Study the drawing (mm; zero at the part's minimum x, y, z) and answer. A direction names the side the tool comes from. Round coordinates to 2 decimals unless told otherwise and drop trailing zeros. Loops run counter-clockwise (first coordinate to the right, second up) from the corner with the lowest first, then second, coordinate; pieces in that order, holes last. Notation, with made-up numbers: M 76.25,72.5 L 90.25,72.5 A22 ccw 90.25,93.5 Z; hole C -12,49 d2. An arc over 180 degrees is marked long. Put each result on its own line as item: value. Start each with the question number.
(1) Which of the six approach directions +Z, -Z, +X, -X, +Y, -Y give full straight-line access (tool end or side, diameter ignored) to the marked faces 4 and 5?
(2) Flat-ended cylindrical pins translate along their axes: P1, Ø3.5, axis at x = 4.5, z = 35.5, coming from the -Y side; P2, Ø13, axis at y = 15, z = 15, coming from the -X side; P3, Ø3.5, axis at x = 4.5, z = 36, coming from the +Y side. Find the tip coordinate at first contact, or state that the pin passes through.
(3) Straight lines are drawn through the part: line 1 (Z direction, x = 4.25, y = 15) (3 decimals); line 2 (Y direction, x = 2.25, z = 15); line 3 (Y direction, x = 3.25, z = 33). For each, find the intervals that lie inside material, in ascending order.
(4) Determine the mould class of the marked faces 1, 2 and 3 for opening direction Z: released by +Z, released by -Z, zero draft, split by the parting line, or undercut.
(5) Section B-B, the plane y = 15 is taken. Determine the outline of the cut face in (x, z) (3 decimals).
(6) Section A-A, the plane z = 15 is taken. Determine the outline of the cut face in (x, y), then the cut area to 3 significant figures.
(7) Section C-C, the plane x = 6.25 is taken. Determine the outline of the cut face in (y, z) (3 decimals), then the cut area to 3 significant figures.
(8) Section D-D, the plane z = 32.5 is taken. Determine the outline of the cut face in (x, y), then the cut area to 3 significant figures.
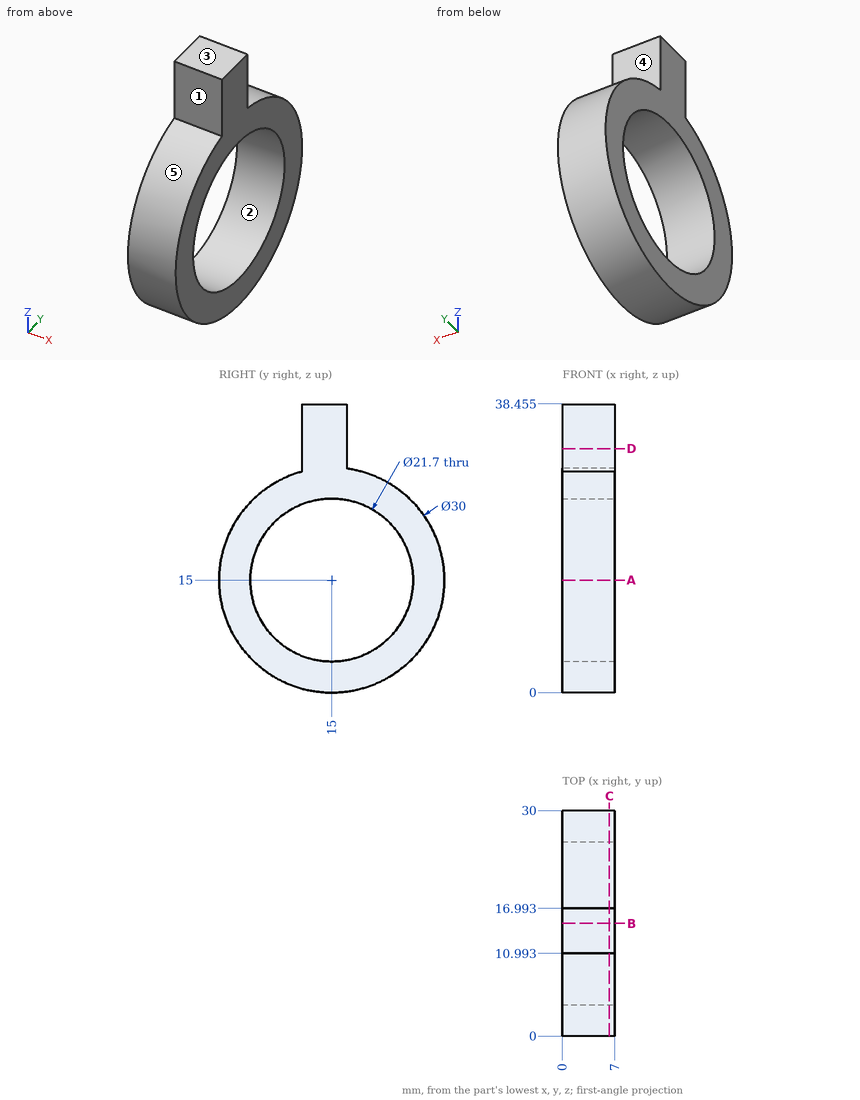
Recorded:
1. face 4: +Z, +X, -X, +Y
1. face 5: +X, -X
2. P1: stops at y = 10.99
2. P2: passes through
2. P3: stops at y = 16.99
3. line 1: z = 0 to 4.15, 25.85 to 38.455
3. line 2: y = 0 to 4.15, 25.85 to 30
3. line 3: y = 10.99 to 16.99
4. face 1: zero draft
4. face 2: undercut
4. face 3: released by +Z
5. outline: M 0,0 L 7,0 L 7,4.15 L 0,4.15 Z; M 0,25.85 L 7,25.85 L 7,38.455 L 0,38.455 Z
6. outline: M 0,0 L 7,0 L 7,4.15 L 0,4.15 Z; M 0,25.85 L 7,25.85 L 7,30 L 0,30 Z
6. area: 58.1 mm²
7. outline: M 10.993,29.455 A15 ccw long 16.993,29.867 L 16.993,38.455 L 10.993,38.455 Z; hole C 15,15 d21.7
7. area: 389 mm²
8. outline: M 0,10.99 L 7,10.99 L 7,16.99 L 0,16.99 Z
8. area: 42.0 mm²
